from build123d import *

# Parameters (mm, degrees)
SKETCH1_W                      = 64.77
SKETCH1_H                      = 50.8
SKETCH1_R                      = 2.5527
SKETCH1_R_2                    = 6.35
BOSS_EXTRUDE1_DEPTH            = 12.7
F_7_0_201_DIAMETER_HOLE1_D     = 5.1054
F_7_0_201_DIAMETER_HOLE1_DEPTH = 70.104
F_7_0_201_DIAMETER_HOLE1_TIP   = 1.533816902
SKETCH6_R                      = 3.9624
CUT_EXTRUDE1_DEPTH             = 4.826
SKETCH7_W                      = 20.32
SKETCH7_H                      = 25.4
CUT_EXTRUDE2_DEPTH             = 49.543247728


with BuildPart() as part:
    # Sketch1 → Boss-Extrude1 (new body)
    with BuildSketch(Plane.XY):
        with Locations((6.985, 0)):
            Rectangle(SKETCH1_W, SKETCH1_H)
        with Locations(Location((-19.05, 19.05, 0), (0, 0, 180))):
            Circle(SKETCH1_R, mode=Mode.SUBTRACT)
        with Locations((19.05, 19.05)):
            Circle(SKETCH1_R, mode=Mode.SUBTRACT)
        with Locations((19.05, -19.05)):
            Circle(SKETCH1_R, mode=Mode.SUBTRACT)
        with Locations((10.16, -19.05)):
            Circle(SKETCH1_R, mode=Mode.SUBTRACT)
        with Locations((14.605, 0)):
            Circle(SKETCH1_R_2, mode=Mode.SUBTRACT)
    extrude(amount=BOSS_EXTRUDE1_DEPTH)

    # #7 (0.201) Diameter Hole1
    with Locations(Plane(origin=(-24.721209515, -12.864288698, 0), x_dir=(1, 0, 0), z_dir=(0, 0, -1))):
        with Locations((57.741209515, 6.185711302), (57.741209515, -31.914288698), (43.771209515, -24.294288698)):
            Hole(F_7_0_201_DIAMETER_HOLE1_D / 2, depth=F_7_0_201_DIAMETER_HOLE1_DEPTH)
            with Locations((0, 0, -(F_7_0_201_DIAMETER_HOLE1_DEPTH + F_7_0_201_DIAMETER_HOLE1_TIP / 2))):  # 118° drill point
                Cone(0, F_7_0_201_DIAMETER_HOLE1_D / 2, F_7_0_201_DIAMETER_HOLE1_TIP, mode=Mode.SUBTRACT)

    # Sketch6 → Cut-Extrude1 (cut)
    with BuildSketch(Plane(origin=(0, 0, 12.7), x_dir=(-1, 0, 0), z_dir=(0, 0, -1))):
        with Locations((-19.05, 19.05)):
            Circle(SKETCH6_R)
        with Locations((-19.05, -19.05)):
            Circle(SKETCH6_R)
        with Locations((-10.16, -19.05)):
            Circle(SKETCH6_R)
        with Locations((19.05, 19.05)):
            Circle(SKETCH6_R)
    extrude(amount=CUT_EXTRUDE1_DEPTH, mode=Mode.SUBTRACT)

    # Sketch7 → Cut-Extrude2 (cut, through all)
    with BuildSketch(Plane(origin=(0, 0, 0), x_dir=(-1, 0, 0), z_dir=(0, 0, -1))):
        with Locations((15.24, -12.7)):
            Rectangle(SKETCH7_W, SKETCH7_H)
    extrude(amount=-CUT_EXTRUDE2_DEPTH, mode=Mode.SUBTRACT)


solid = part.part
Input: part model. Units: mm. Frame: model coordinates. A direction names the side the tool comes from. Coordinates: 2 decimals unless noted, no trailing zeros. Loops run counter-clockwise (first coordinate to the right, second up) from the corner with the lowest first, then second, coordinate; pieces in that order, holes last. Notation, with made-up numbers: (54.25, -5.75) -> (100.25, -5.75) arc R30 ccw to (100.25, 30.25) -> close; hole circle Ø9 at (69.5, -34). An arc over 180 degrees is marked (long way). Write each question's results on one line, items separated by ' | '. Start each with the question number.
Q1. Pin query (flat end, axial travel): pin 1 (2.5 mm diameter, centred on x = 9, y = -17.5, fed in from +Z); pin 2 (4 mm diameter, centred on y = -17, z = 8.5, fed in from -X). Return the tip coordinate at first contact, or that it passes through.
Q2. Ray query, line 1 (X direction, y = 20, z = 7.75); line 2 (Y direction, x = 34, z = 3); line 3 (Y direction, x = -19.05, z = 2.25). Return the intervals inside material, ascending. Write a range as from..to.
Q3. Section A-A, the plane y = 11.43. Return the cut outline in (x, z).
Q4. Section B-B, the plane x = 33.02. Return the cut outline in (y, z), plus the area to 3 significant figures.
Q5. Pull-direction query (X, two-part tool) for faces 3 (the flat face through (-15, 0, 6)), 4 (the flat face through (16, -19, 7.874)), 5 (the flat face through (-5.08, -13, 6)); classes: released by +X, released by -X, zero draft, split by the parting line, or undercut.
Q6. Section D-D, the plane y = -19.05. Return the cut outline in (x, z), plus the area to 3 significant figures.
Q7. Reachability of faces 1 (the flat face through (10, -22, 7.874)), 2 (the flat face through (7, 0, 12.7)) from +Z, -Z, +X, -X, +Y, -Y: full face, straight path, thin tool, end or side. Return the list, or none.
Q8. Section C-C, the plane x = -19.05. Return the cut outline in (y, z).
Found:
1) pin 1: z = 7.87 | pin 2: x = -5.08
2) line 1: -25.4..-21.42, -16.68..16.68, 21.42..30.65, 35.39..39.37 | line 2: -25.4..-21.41, -16.69..16.69, 21.41..25.4 | line 3: 0..16.5, 21.6..25.4
3) outline: (-25.4, 0) -> (16.5, 0) -> (16.5, 12.7) -> (-25.4, 12.7) -> close; (21.6, 0) -> (39.37, 0) -> (39.37, 12.7) -> (21.6, 12.7) -> close
4) outline: (-25.4, 0) -> (-21.6, 0) -> (-21.6, 12.7) -> (-25.4, 12.7) -> close; (-16.5, 0) -> (16.5, 0) -> (16.5, 12.7) -> (-16.5, 12.7) -> close; (21.6, 0) -> (25.4, 0) -> (25.4, 12.7) -> (21.6, 12.7) -> close | area: 515 mm2
5) face 3: zero draft | face 4: undercut | face 5: released by -X
6) outline: (-5.08, 0) -> (7.61, 0) -> (7.61, 7.87) -> (6.2, 7.87) -> (6.2, 12.7) -> (-5.08, 12.7) -> close; (12.71, 0) -> (16.5, 0) -> (16.5, 7.87) -> (15.09, 7.87) -> (15.09, 12.7) -> (14.12, 12.7) -> (14.12, 7.87) -> (12.71, 7.87) -> close; (21.6, 0) -> (30.47, 0) -> (30.47, 12.7) -> (23.01, 12.7) -> (23.01, 7.87) -> (21.6, 7.87) -> close; (35.57, 0) -> (39.37, 0) -> (39.37, 12.7) -> (35.57, 12.7) -> close | area: 343 mm2
7) face 1: +Z | face 2: +Z, +X, -X, +Y, -Y
8) outline: (0, 0) -> (16.5, 0) -> (16.5, 7.87) -> (15.09, 7.87) -> (15.09, 12.7) -> (0, 12.7) -> close; (21.6, 0) -> (25.4, 0) -> (25.4, 12.7) -> (23.01, 12.7) -> (23.01, 7.87) -> (21.6, 7.87) -> close
